Check sheet for the modelled part. Datum: model origin and axes. Units: mm. Face numbers are marked on the shaded views. A direction names the side the tool comes from. Coordinates: 2 decimals unless noted, no trailing zeros. Loops run counter-clockwise (first coordinate to the right, second up) from the corner with the lowest first, then second, coordinate; pieces in that order, holes last.
Autodesk Inventor part; units mm, degrees
ref_plane "YZ Plane" through (0, 0, 0) normal (1, 0, 0) x (0, 1, 0)
ref_plane "XZ Plane" through (0, 0, 0) normal (0, 1, 0) x (-1, 0, 0)
ref_plane "XY Plane" through (0, 0, 0) normal (0, 0, 1) x (1, 0, 0)
sketch "Sketch1" plane through (0, 0, 0) normal (0, 1, 0) x (-1, 0, 0)
  line L0 (0, -55.88) -> (-12.7, -55.88)
  line L1 (-12.7, 0) -> (0, 0)
  line L2 (0, 0) -> (0, -20.94)
  line L3 (0, -34.94) -> (0, -55.88)
  line L4 (-12.7, -55.88) -> (-12.7, -34.94)
  line L5 (-12.7, -20.94) -> (-12.7, 0)
  line L6 (0, -20.94) -> (0, -34.94)
  line L7 (-12.7, -20.94) -> (-12.7, -34.94)
  dimension "d1" = 55.88
  dimension "d2" = 12.7
extrude "Extrusion1" add sketch "Sketch1" along normal blind 1.5
sketch "Sketch2" plane through (0, 1.5, 0) normal (0, 1, 0) x (1, 0, 0)
  line L0 (12.7, 0) -> (12.7, 55.88)
  line L1 (12.7, 0) -> (10.16, 0)
  line L2 (12.7, 2.54) -> (12.7, 0)
  circle A0 centre (10.16, 2.54) radius 1.092
  circle A1 centre (10.16, 53.34) radius 1.092
  point P0 (0, 0)
  dimension "d8" = 2.184
  dimension "d10" = 2.184
extrude "Extrusion2" cut sketch "Sketch2" against normal blind 1.5
sketch "Sketch5" plane through (0, 0, 0) normal (0, 0, 1) x (1, 0, 0)
  line L0 (12.7, 0) -> (0, 0)
  line L1 (6.35, 0) -> (6.35, 1.5)
  line L2 (12.7, 1.5) -> (0, 1.5)
  line L3 (0, 0) -> (0, 1.5)
  line L4 (0, 0.75) -> (12.7, 0.75)
  line L5 (12.7, 0) -> (12.7, 1.5)
  circle A0 centre (6.35, 0.75) radius 5.175
  dimension "d30" = 10.35
extrude "Extrusion5" add sketch "Sketch5" along normal blind 2 contours A0 L0 | L0 L1 L4 A0 | L0 A0 L4 L1 | L4 L1 L2 A0 | L4 A0 L2 L1 | L2 A0
sketch "Sketch6" plane through (6.35, 0.75, 2) normal (0, 0, 1) x (1, 0, 0)
  circle A0 centre (0, 0) radius 5.175
  circle A1 centre (0, 0) radius 3.175
  point P0 (-6.35, -0.75)
  dimension "d35" = 6.35
extrude "Extrusion6" add sketch "Sketch6" along normal blind 9
sketch "Sketch7" plane through (12.7, 0, -55.88) normal (0, 0, -1) x (-1, 0, 0)
  line L0 (0, 0) -> (0, 1.5)
  line L1 (0, 0.75) -> (12.7, 0.75)
  line L2 (12.7, 0) -> (12.7, 1.5)
  line L3 (11.4704, 1.5) -> (1.2296, 1.5)
  line L4 (6.35, 1.5) -> (6.35, 0)
  circle A0 centre (6.35, 0.75) radius 5.175
extrude "Extrusion7" add sketch "Sketch7" along normal blind 2
sketch "Sketch8" plane through (6.35, 0.75, -57.88) normal (0, 0, -1) x (-1, 0, 0)
  circle A0 centre (0, 0) radius 5.175
  circle A1 centre (0, 0) radius 3.175
  point P0 (6.35, -0.75)
  dimension "d40" = 6.35
extrude "Extrusion8" add sketch "Sketch8" along normal blind 9
thread "Thread1"
thread "Thread2"
sketch "Sketch9" plane through (0, 0, 0) normal (0, 0, -1) x (-1, 0, 0)
  arc A0 (-11.4704, 0) -> (-1.2296, 0) centre (-6.35, 0.75) ccw
  line L0 (0, 0) -> (-1.2296, 0)
  line L1 (-11.4704, 0) -> (-1.2296, 0)
  circle A1 centre (-6.35, 0.75) radius 5.175
extrude "Extrusion9" add sketch "Sketch9" along normal up to next contours L1 A0
sketch "Sketch10" plane through (10.16, 0, -2.54) normal (0, 1, 0) x (1, 0, 0)
  circle A0 centre (0, 0) radius 1.092
  circle A1 centre (0, 50.8) radius 1.092
  circle A2 centre (0, 50.8) radius 1.092
  point P0 (-10.16, -2.54)
  dimension "d60" = 2.184
extrude "Extrusion10" cut sketch "Sketch10" against normal up to next
sketch "Sketch12" plane through (0, 1.5, 0) normal (0, 1, 0) x (1, 0, 0)
  circle A0 centre (10.16, 2.54) radius 1.092
  circle A1 centre (10.16, 2.54) radius 1.092
  circle A2 centre (10.16, 2.54) radius 2.2225
  circle A3 centre (10.16, 53.34) radius 1.092
  circle A4 centre (10.16, 53.34) radius 1.092
  circle A5 centre (10.16, 53.34) radius 2.2225
  point P0 (0, 0)
  dimension "d54" = 4.445
  dimension "d55" = 4.445
extrude "Extrusion11" cut sketch "Sketch12" against normal blind 5.925
sketch "Sketch13" plane through (0, 1.5, 0) normal (0, 1, 0) x (1, 0, 0)
  line L0 (12.7, 0) -> (12.7, 55.88)
  line L1 (12.7, 55.88) -> (0, 55.88)
  line L2 (0, 55.88) -> (0, 0)
  line L3 (0, 0) -> (12.7, 0)
  line L4 (12.7, 0) -> (12.7, 55.88)
  circle A0 centre (10.16, 53.34) radius 1.092
  circle A1 centre (10.16, 53.34) radius 1.092
  circle A2 centre (10.16, 2.54) radius 1.092
  circle A3 centre (10.16, 2.54) radius 1.092
extrude "Extrusion12" add sketch "Sketch13" along normal blind 10.4375
thread "Thread5"
thread "Thread6"
sketch "Sketch14" plane through (10.16, 1.5, -53.34) normal (0, -1, 0) x (1, 0, 0)
  circle A0 centre (0, 0) radius 1.092
  circle A1 centre (0, 0) radius 2.2225
  circle A2 centre (0, 50.8) radius 2.2225
  circle A3 centre (0, 50.8) radius 2.2225
  circle A4 centre (0, 0) radius 1.092
  circle A5 centre (0, 50.8) radius 1.092
  point P0 (-10.16, 53.34)
extrude "Extrusion13" cut sketch "Sketch14" against normal blind 1
sketch "Sketch15" plane through (0, 11.9375, 0) normal (0, 1, 0) x (1, 0, 0)
  line L0 (12.7, 0) -> (12.7, 6.985)
  line L1 (12.7, 0) -> (12.7, 55.88)
  line L2 (12.7, 0) -> (19.685, 0) construction
  line L3 (11.525, -11) -> (11.525, 66.88)
  line L4 (11.43, 6.985) -> (13.97, 6.985) construction
  line L5 (11.43, 6.985) -> (12.43, 6.985) construction
  line L6 (11.43, 9.525) -> (12.43, 9.525) construction
  line L7 (12.7, 5.985) -> (12.7, 10.525)
  line L8 (12.7, 5.985) -> (12.7, 5.485)
  line L9 (12.7, 5.485) -> (9.93, 5.485)
  line L10 (9.93, 5.485) -> (9.93, 11.025)
  line L11 (9.93, 11.025) -> (12.7, 11.025)
  line L12 (12.7, 11.025) -> (12.7, 10.525)
  point P0 (0, 0)
  dimension "d72" = 90
  dimension "d130" = 0.5
  dimension "d131" = 2.77
  dimension "d132" = 5.54
extrude "Extrusion14" cut sketch "Sketch15" against normal blind 8
sketch "Sketch16" plane through (0, 11.9375, 0) normal (0, 1, 0) x (1, 0, 0)
  line L0 (12.7, 0) -> (12.7, 55.88)
  line L1 (12.7, 40.234) -> (13.97, 40.234) construction
  line L2 (0, 0) -> (12.7, 0)
  line L3 (11.43, 0) -> (40.005, 0) construction
  line L4 (11.525, -11) -> (11.525, 66.88)
  line L5 (11.43, 28.575) -> (13.97, 28.575) construction
  line L6 (11.43, 46.355) -> (12.43, 46.355) construction
  line L7 (11.43, 28.575) -> (13.97, 28.575) construction
  line L8 (11.43, 20.955) -> (12.43, 20.955) construction
  line L9 (6.89, 19.955) -> (6.89, 47.355)
  line L10 (12.7, 47.355) -> (12.7, 19.955)
  line L11 (6.89, 47.355) -> (6.89, 47.855)
  line L12 (6.89, 47.855) -> (12.7, 47.855)
  line L13 (12.7, 47.855) -> (12.7, 47.355)
  line L14 (12.7, 19.955) -> (12.7, 19.455)
  line L15 (12.7, 0) -> (12.7, 55.88)
  line L16 (12.7, 19.455) -> (6.89, 19.455)
  line L17 (6.89, 19.455) -> (6.89, 19.955)
  point P0 (12.7, 10.525)
  dimension "d123" = 5.81
  dimension "d129" = 28.4
extrude "Extrusion15" cut sketch "Sketch16" against normal blind 8 contours L16 L4 L12 L0 | L16 L17 L9 L11 L12 L4
properties part number "Line Sensor 6 Bracket"
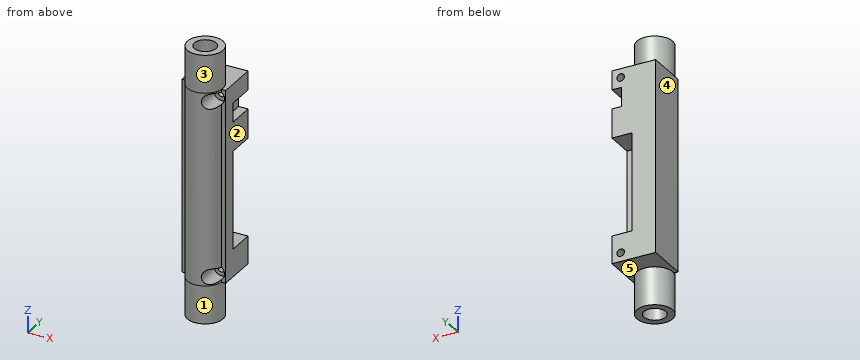
1) Section check D-D on z = 6.5. Enter the section's corners in (x, y) (3 decimals), plus the area to 3 significant figures.
Answer sheet:
outline: circle Ø10.35 at (6.35, 0.75); hole circle Ø6.35 at (6.35, 0.75)
area: 52.5 mm2
2) Depth check by flat-ended pin: pin 1 (2 mm diameter, centred on x = 10.5, z = -53.5, fed in from -Y); pin 2 (6 mm diameter, centred on x = 7, y = 0, fed in from -Z); pin 3 (1 mm diameter, centred on x = 5, z = 1.5, fed in from -Y); pin 4 (1.9 mm diameter, centred on x = 7.5, y = 0.5, fed in from -Z). Enter the tip coordinate at first touch or a pass-through.
Answer sheet:
pin 1: stops at y = 2.5
pin 2: stops at z = -66.88
pin 3: stops at y = -4.35
pin 4: stops at z = -57.88
3) Scan lines: line 1 (Z direction, x = 10.16, y = -1.25); line 2 (Z direction, x = 10, y = 3.5); line 3 (Z direction, x = 7.5, y = 5) (3 decimals). Record each from-to range of solid material in increasing order.
Answer sheet:
line 1: z = -66.88 to -55.56, -51.12 to -4.76, -0.32 to 11
line 2: z = -66.88 to -54.42, -52.26 to -3.62, -1.46 to 11
line 3: z = -66.88 to -47.855, -19.455 to 11
4) Section check A-A on y = 0.75. Enter the section's corners in (x, z) (1 decimal).
Answer sheet:
outline: (0, -55.9) - (1.2, -55.9) - (1.2, -66.9) - (3.2, -66.9) - (3.2, -57.9) - (9.5, -57.9) - (9.5, -66.9) - (11.5, -66.9) - (11.5, -55.9) - (12.7, -55.9) - (12.7, 0) - (11.5, 0) - (11.5, 11) - (9.5, 11) - (9.5, 2) - (3.2, 2) - (3.2, 11) - (1.2, 11) - (1.2, 0) - (0, 0) - close; hole circle Ø4.4 at (10.2, -53.3); hole circle Ø4.4 at (10.2, -2.5)
5) Section check B-B on z = -53.34. Enter the section's corners in (x, y), plus the area to 3 significant figures.
Answer sheet:
outline: (0, 0) - (1.23, 0) arc R5.18 ccw to (7.94, -4.18) - (7.94, 2.5) - (9.07, 2.5) - (9.07, 11.94) - (0, 11.94) - close; (11.25, 2.5) - (12.38, 2.5) - (12.38, 0) - (12.7, 0) - (12.7, 11.94) - (11.25, 11.94) - close
area: 144 mm2
6) Section check C-C on y = 7.5. Enter the section's corners in (x, z) (3 decimals).
Answer sheet:
outline: (0, -55.88) - (12.7, -55.88) - (12.7, -47.855) - (6.89, -47.855) - (6.89, -19.455) - (12.7, -19.455) - (12.7, -11.025) - (9.93, -11.025) - (9.93, -5.485) - (12.7, -5.485) - (12.7, 0) - (0, 0) - close; hole circle Ø2.184 at (10.16, -53.34); hole circle Ø2.184 at (10.16, -2.54)
7) Set-up check for the marked faces 1, 2, 3, 4 and 5: record each of +Z, -Z, +X, -X, +Y, -Y from which the full face is reachable in a straight line by a thin tool's end or side.
Answer sheet:
face 1: -Z
face 2: +Z, -Z, +X, +Y, -Y
face 3: +Z
face 4: +Z, -Z, -X, +Y, -Y
face 5: -Z, +Y
